Drawing for the job (mm, zero at the part's lowest x, y, z). Give positions to 0.01 mm unless a question says otherwise; leave off trailing zeros. Order: outer loops, then holes, each group sorted by start corner. A loop starts at its lowest first (then second) coordinate and runs counter-clockwise, first axis right, second up. Notation, with made-up numbers: (18, -1) -> (24, -1) arc R26 cw to (24, 28) -> close; hole circle Ø5 at (64, -5). An arc over 180 degrees is marked (long way). Use one line per item in the form item = value. Start each with the question number.
1) Drop flat-ended pins along their axis: P1, Ø4, axis at y = 13, z = 102, coming from the -X side; P2, Ø2, axis at x = 16, z = 108, coming from the +Y side; P3, Ø1.5, axis at x = 14, z = 30.5, coming from the -Y side; P4, Ø4, axis at y = 8, z = 16.5, coming from the +X side. Give the stop position or say it passes through.
2) Probe line 1 (Z direction, x = 85, y = 3); line 2 (Z direction, x = 86, y = 2.5). List the from-to ranges inside material, lowest first.
3) Cut at D-D, the plane x = 103.5. Give the cut face in (y, z).
4) Cut at B-B, the plane z = 85. Give the cut face in (x, y), and give its area (3 significant figures).
5) Cut at C-C, the plane x = 85. Give the cut face in (y, z), and give its area (3 significant figures).
6) Cut at A-A, the plane y = 12.75. Give the cut face in (x, z), and give its area (3 significant figures).
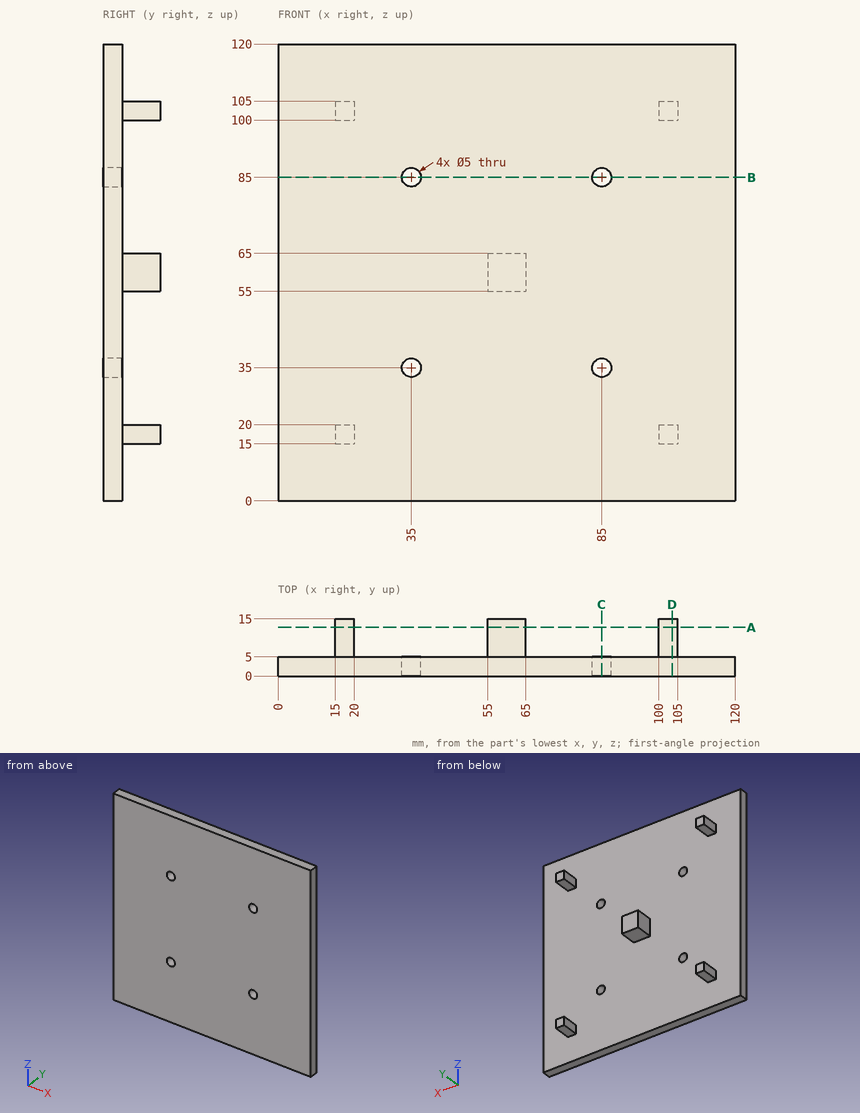
Result:
q1.P1 = 15
q1.P2 = 5
q1.P3 = 0
q1.P4 = 105
q2.line_1 = 0 to 32.5, 37.5 to 82.5, 87.5 to 120
q2.line_2 = 0 to 32.71, 37.29 to 82.71, 87.29 to 120
q3.outline = (0, 0) -> (5, 0) -> (5, 15) -> (15, 15) -> (15, 20) -> (5, 20) -> (5, 100) -> (15, 100) -> (15, 105) -> (5, 105) -> (5, 120) -> (0, 120) -> close
q4.outline = (0, 0) -> (32.5, 0) -> (32.5, 5) -> (0, 5) -> close; (37.5, 0) -> (82.5, 0) -> (82.5, 5) -> (37.5, 5) -> close; (87.5, 0) -> (120, 0) -> (120, 5) -> (87.5, 5) -> close
q4.area = 550 mm²
q5.outline = (0, 0) -> (5, 0) -> (5, 32.5) -> (0, 32.5) -> close; (0, 37.5) -> (5, 37.5) -> (5, 82.5) -> (0, 82.5) -> close; (0, 87.5) -> (5, 87.5) -> (5, 120) -> (0, 120) -> close
q5.area = 550 mm²
q6.outline = (15, 15) -> (20, 15) -> (20, 20) -> (15, 20) -> close; (15, 100) -> (20, 100) -> (20, 105) -> (15, 105) -> close; (55, 55) -> (65, 55) -> (65, 65) -> (55, 65) -> close; (100, 15) -> (105, 15) -> (105, 20) -> (100, 20) -> close; (100, 100) -> (105, 100) -> (105, 105) -> (100, 105) -> close
q6.area = 200 mm²
